CAD build for the part. Positions are in the model's coordinates, mm. Give positions to 0.01 mm unless a question says otherwise; leave off trailing zeros. Order: outer loops, then holes, each group sorted by start corner. A loop starts at its lowest first (then second) coordinate and runs counter-clockwise, first axis right, second up.
```python
from build123d import *

# Parameters (mm, degrees)
SKETCH1_W           = 538.9562500000001
SKETCH1_H           = 323.84999999999997
BOSS_EXTRUDE1_DEPTH = 9.525
BOSS_EXTRUDE2_DEPTH = 538.95625
BOSS_EXTRUDE3_DEPTH = 538.95625
CUT_EXTRUDE1_DEPTH  = 317.16786663403565
FILLET1_R           = 19.05
SKETCH6_W           = 526.3492063472065
SKETCH6_H           = 297.32296140336337
CUT_EXTRUDE2_DEPTH  = 0.0254


with BuildPart() as part:
    # Sketch1 → Boss-Extrude1 (new body)
    with BuildSketch(Plane.XY):
        Rectangle(SKETCH1_W, SKETCH1_H)
    extrude(amount=BOSS_EXTRUDE1_DEPTH)

    # Sketch3 → Boss-Extrude2 (add)
    with BuildSketch(Plane(origin=(269.47812500000003, 0, 0), x_dir=(0, 0, -1), z_dir=(1, 0, 0))):
        Polygon((-9.525, 161.92499999999998), (0.253999999999999, 161.92499999999998), (8.062497413649258, -161.92499999999998), (0, -161.92499999999998), (-9.525, -161.92499999999998), (-11.952702586350743, -161.92499999999998), (-11.95270258635074, -142.5194), (-9.525, -142.5194), align=None)
    extrude(amount=-BOSS_EXTRUDE2_DEPTH)

    # Sketch4 → Boss-Extrude3 (add)
    with BuildSketch(Plane(origin=(269.47812500000003, 0, 0), x_dir=(0, 0, -1), z_dir=(1, 0, 0))):
        Polygon((37.193592332721494, 78.37169999999999), (36.576258201765725, -80.3770996759999), (6.157552828059534, -82.9192359761992), (2.191447852529644, 81.57119390858017), align=None)
    extrude(amount=-BOSS_EXTRUDE3_DEPTH)

    # Sketch5 → Cut-Extrude1 (cut, through all)
    with BuildSketch(Plane(origin=(0, 0.10020320699075866, -4.1558326608693195), x_dir=(-1, 0, 0), z_dir=(0, 0.024104457676112176, -0.9997094453490677))):
        Polygon((-139.684125, -83.04356787806702), (-139.68412500000005, 81.4946693567972), (-269.47812500000003, 81.49466935679719), (-269.47812500000003, -83.04356787806695), align=None)
        Polygon((269.47812500000003, 81.4946693567972), (139.71587499999993, 81.49466935679719), (139.71587499999995, -83.04356787806701), (269.47812500000003, -83.04356787806702), align=None)
    extrude(amount=CUT_EXTRUDE1_DEPTH, mode=Mode.SUBTRACT)

    # Fillet1
    fillet1_edges = [part.edges().sort_by_distance(p)[0] for p in [
        (-0.01587499999999409, -82.9192359761992, -6.157552828059534),
        (-0.01587499999993724, 81.57119390858017, -2.191447852529644),
        (139.68412500000002, -0.6740210338095626, -4.17450034029459),
        (-139.71587499999993, -0.6740210338095626, -4.17450034029459),
    ]]
    fillet(fillet1_edges, radius=FILLET1_R)

    # Sketch6 → Cut-Extrude2 (cut)
    with BuildSketch(Plane.XY.offset(9.525)):
        with Locations((2.842e-14, 9.70280000000001)):
            Rectangle(SKETCH6_W, SKETCH6_H)
    extrude(amount=-CUT_EXTRUDE2_DEPTH, mode=Mode.SUBTRACT)


solid = part.part
```
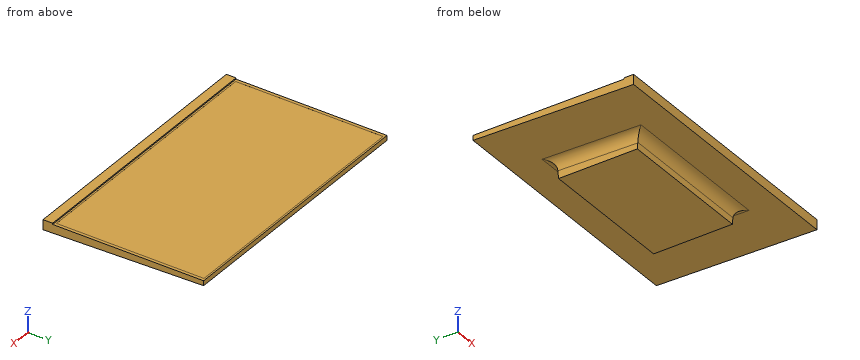
Item 1: Drop flat-ended pins along their axis: pin 1 Ø6 at (x, z) = (-77.5, -26.5) entering from +Y; pin 2 Ø6 at (y, z) = (0, -20.5) entering from +X; pin 3 Ø6 at (x, y) = (13, 105.5) entering from -Z. Give the stop position or say it passes through.
Item 2: Wall check: L1, parallel to Z at x = 80.5, y = 99; L2, parallel to X at y = -43, z = -22; L3, parallel to X at y = -40.5, z = -33.5. Give the ranges that are in metal, low to high.
Item 3: Slice it at B-B (y = 115). Give the cut face in (x, z) (3 decimals).
Item 4: Slice it at C-C (z = -31.5). Give the cut face in (x, y), and give its area (3 significant figures).
A:
1. pin 1: stops at y = 79.62
1. pin 2: stops at x = 140.56
1. pin 3: stops at z = -1.69
2. L1: z = -1.77 to 9.5
2. L2: x = -139.85 to 139.82
2. L3: x = -139.72 to 139.68
3. outline: (-269.478, -1.385) - (269.478, -1.385) - (269.478, 9.525) - (263.175, 9.525) - (263.175, 9.5) - (-263.175, 9.5) - (-263.175, 9.525) - (-269.478, 9.525) - close
4. outline: (-139.72, -80.8) - (139.68, -80.8) - (139.68, 78.89) - (-139.72, 78.89) - close
4. area: 44,600 mm2
